The model under review builds one solid part; all positions refer to its coordinate system, in mm. Face numbers are marked on the shaded views. A direction names the side the tool comes from. Round coordinates to 2 decimals unless told otherwise and drop trailing zeros. Write each loop counter-clockwise with the first axis right and the second up, starting at its lowest first coordinate (ties: lowest second). Pieces come first, ordered by that corner, then holes.
Item 1: Add section B-B (x = 6). Give the boundary of the cut face in (y, z) (3 decimals), plus the area to 3 significant figures.
Item 2: To check wall thickness, follow L1, parallel to Z at x = 7.5, y = -7.55; L2, parallel to Z at x = 7.5, y = -8.7; L3, parallel to X at y = -9.75, z = 6.24. State the ranges of each line that lie inside material, in increasing order.
Item 3: Add section A-A (y = -8.75). Give the boundary of the cut face in (x, z), plus the area to 3 significant figures.
Item 4: Machinability: for the marked faces 1, 2, 3, 4 and 5, which of the approach directions +Z, -Z, +X, -X, +Y, -Y give a long, thin tool a straight path to every point of the face, cutting with its end or side? Answer none if there is none.
Item 5: Add section D-D (y = -6.5). Give the boundary of the cut face in (x, z).
Item 6: Clearance check with flat-ended pins moving along their axes: pin 1 Ø1.5 at (y, z) = (-9, 5.5) entering from +X; pin 2 Ø1.5 at (x, z) = (10.5, 0) entering from -Y; pin 3 Ø2 at (x, z) = (8.5, -8.5) entering from +Y. State where each tip first meets the part, or that it passes through.
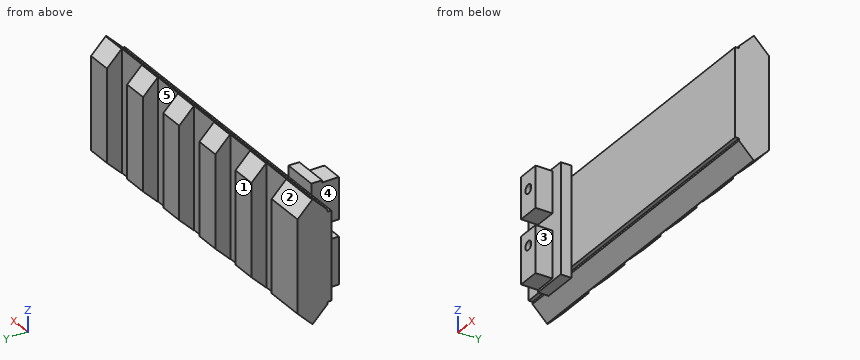
```python
from build123d import *

# Parameters (mm, degrees)
BOSS_EXTRUDE1_DEPTH             = 57
SKETCH2_W                       = 5.57
SKETCH2_H                       = 21.59
CUT_EXTRUDE1_DEPTH              = 2.667
LPATTERN1_COUNT                 = 5
LPATTERN1_PITCH                 = 9.97
SKETCH4_W                       = 6.3
SKETCH4_H                       = 19.5
BOSS_EXTRUDE3_DEPTH             = 1.9
SKETCH3_W                       = 4
SKETCH3_H                       = 8.35
SKETCH3_H_2                     = 7.35
BOSS_EXTRUDE2_DEPTH             = 3
TAP_DRILL_FOR_M2X0_4_TAP1_D     = 1.6
TAP_DRILL_FOR_M2X0_4_TAP1_DEPTH = 5.233
TAP_DRILL_FOR_M2X0_4_TAP1_TIP   = 0.480688495


with BuildPart() as part:
    # Sketch1 → Boss-Extrude1 (new body)
    with BuildSketch(Plane(origin=(0, 0, 0), x_dir=(0, 0, -1), z_dir=(1, 0, 0))):
        Polygon((-7.8359, -6), (7.8359, -6), (7.8359, -5.334), (8.2042, -5.334), (10.795, -2.7432), (10.795, -2.5908), (8.2042, 0), (-8.2042, 0), (-10.795, -2.5908), (-10.795, -2.7432), (-8.2042, -5.334), (-7.8359, -5.334), align=None)
    extrude(amount=BOSS_EXTRUDE1_DEPTH)

    # Sketch2 → Cut-Extrude1 (cut)
    with BuildSketch(Plane(origin=(0, 0, 0), x_dir=(1, 0, 0), z_dir=(0, 1, 0))):
        with Locations((49.815, 0)):
            Rectangle(SKETCH2_W, SKETCH2_H)
    cut_extrude1 = extrude(amount=-CUT_EXTRUDE1_DEPTH, mode=Mode.SUBTRACT)

    # LPattern1: Cut-Extrude1 ×5
    with Locations(*[(-i * LPATTERN1_PITCH, 0, 0) for i in range(1, LPATTERN1_COUNT)]):
        add(cut_extrude1, mode=Mode.SUBTRACT)

    # Sketch4 → Boss-Extrude3 (add)
    with BuildSketch(Plane.XZ.offset(6)):
        with Locations((8.65, 0)):
            Rectangle(SKETCH4_W, SKETCH4_H)
    extrude(amount=BOSS_EXTRUDE3_DEPTH)

    # Sketch3 → Boss-Extrude2 (add)
    with BuildSketch(Plane.XZ.offset(7.9)):
        with Locations((7.5, -5.165)):
            Rectangle(SKETCH3_W, SKETCH3_H)
        with Locations((7.5, 5.665)):
            Rectangle(SKETCH3_W, SKETCH3_H_2)
    extrude(amount=BOSS_EXTRUDE2_DEPTH)

    # Tap Drill for M2x0.4 Tap1
    with Locations(Plane(origin=(0, -10.9, 0), x_dir=(-1, 0, 0), z_dir=(0, -1, 0))):
        with Locations((-7.5, -6.24), (-7.5, 3.56)):
            Hole(TAP_DRILL_FOR_M2X0_4_TAP1_D / 2, depth=TAP_DRILL_FOR_M2X0_4_TAP1_DEPTH)
            with Locations((0, 0, -(TAP_DRILL_FOR_M2X0_4_TAP1_DEPTH + TAP_DRILL_FOR_M2X0_4_TAP1_TIP / 2))):  # 118° drill point
                Cone(0, TAP_DRILL_FOR_M2X0_4_TAP1_D / 2, TAP_DRILL_FOR_M2X0_4_TAP1_TIP, mode=Mode.SUBTRACT)


solid = part.part
```
Numbers:
1. outline: (-10.9, -9.34) - (-7.9, -9.34) - (-7.9, -9.75) - (-6, -9.75) - (-6, -7.836) - (-5.334, -7.836) - (-5.334, -8.204) - (-2.743, -10.795) - (-2.591, -10.795) - (0, -8.204) - (0, 8.204) - (-2.591, 10.795) - (-2.743, 10.795) - (-5.334, 8.204) - (-5.334, 7.836) - (-6, 7.836) - (-6, 9.75) - (-7.9, 9.75) - (-7.9, 9.34) - (-10.9, 9.34) - (-10.9, 1.99) - (-7.9, 1.99) - (-7.9, -0.99) - (-10.9, -0.99) - close
1. area: 196 mm2
2. L1: z = -9.75 to -4.36, -2.76 to 5.44, 7.04 to 9.75
2. L2: z = -9.34 to -4.36, -2.76 to -0.99, 1.99 to 5.44, 7.04 to 9.34
2. L3: x = 5.5 to 6.7, 8.3 to 9.5
3. outline: (5.5, -9.34) - (9.5, -9.34) - (9.5, -0.99) - (5.5, -0.99) - close; (5.5, 1.99) - (9.5, 1.99) - (9.5, 9.34) - (5.5, 9.34) - close; hole circle Ø1.6 at (7.5, -3.56); hole circle Ø1.6 at (7.5, 6.24)
3. area: 58.8 mm2
4. face 1: +Z, -Z, +X, -X, +Y
4. face 2: +Z, +X, -X, +Y
4. face 3: +Z, -Z, +X, -Y
4. face 4: +Z, -Z, -X, -Y
4. face 5: +Z, -Z, +Y
5. outline: (5.5, -9.75) - (11.8, -9.75) - (11.8, 9.75) - (5.5, 9.75) - close; hole circle Ø1.6 at (7.5, -3.56); hole circle Ø1.6 at (7.5, 6.24)
6. pin 1: stops at x = 9.5
6. pin 2: stops at y = -7.9
6. pin 3: stops at y = -2.67
